Geometry check sheet. Reference: the model listing, model coordinates, mm. Coordinates: 2 decimals unless noted, no trailing zeros. Loops run counter-clockwise (first coordinate to the right, second up) from the corner with the lowest first, then second, coordinate; pieces in that order, holes last. Notation, with made-up numbers: M -21.5,7 L 28.5,7 A9 cw 28.5,24 Z; hole C -4,48.25 d9. An arc over 180 degrees is marked long. Use CSV: the item, a comma, the result in double quotes.
```python
from build123d import *

# Parameters (mm, degrees)
EXTRUDE_1_DEPTH     = 100
SKETCH_2_R          = 1.45
CUT_EXTRUDE_1_DEPTH = 10
SKETCH_3_R          = 1.45
CUT_EXTRUDE_2_DEPTH = 10


with BuildPart() as part:
    # Эскиз1 → Бобышка-Вытянуть1 (new, symmetric)
    with BuildSketch(Plane(origin=(0, 0, 0), x_dir=(0, 0, -1), z_dir=(1, 0, 0))):
        with BuildLine():
            Line((-3.085485457, 17.498657575), (-2.386593122, 13.535042182))
            Line((-2.386593122, 13.535042182), (2.386593122, 13.535042182))
            Line((2.386593122, 13.535042182), (3.085485457, 17.498657575))
            ThreePointArc((3.085485457, 17.498657575), (0, 17.604562424), (-3.085485457, 17.498657575))
        make_face()
    extrude(amount=EXTRUDE_1_DEPTH, both=True)

    # Эскиз2 → Вырез-Вытянуть1 (cut)
    with BuildSketch(Plane(origin=(100, 0, 0), x_dir=(0, 0, -1), z_dir=(1, 0, 0))):
        with Locations((0, 15.604562424)):
            Circle(SKETCH_2_R)
    cut_extrude_1 = extrude(amount=-CUT_EXTRUDE_1_DEPTH, mode=Mode.SUBTRACT)

    # Зеркальное отражение1: Вырез-Вытянуть1 across plane
    add(cut_extrude_1.mirror(Plane(origin=(0, 0, 0), x_dir=(0, 0, 1), z_dir=(1, 0, 0))), mode=Mode.SUBTRACT)

    # Эскиз3 → Вырез-Вытянуть2 (cut)
    with BuildSketch(Plane.XZ.offset(-13.535042182)):
        with Locations(Location((-20, 0, 0), (0, 0, 270))):
            Circle(SKETCH_3_R)
        with Locations(Location((20, 0, 0), (0, 0, 270))):
            Circle(SKETCH_3_R)
    extrude(amount=-CUT_EXTRUDE_2_DEPTH, mode=Mode.SUBTRACT)


solid = part.part
```
1. Section check B-B, the plane x = 35. Record the cut outline in (y, z).
The answers:
outline,"M 13.54,-2.39 L 17.5,-3.09 A45 ccw 17.5,3.09 L 13.54,2.39 Z"
2. Release check for a two-part mould opening along Z. For faces 1 (the flat face through (1.4, 15.54, 2.74)), 2 (the flat face through (1, 13.535, 0)), 3 (the flat face through (1.4, 15.49, -2.73)), 4 (the cylindrical face through (1.4, 17.605, -0.043)) record: +Z half, -Z half, draft (parallel to the pull), parting line (faces both ways), or undercut.
The answers:
face 1,"+Z half"
face 2,"draft"
face 3,"-Z half"
face 4,"parting line"
3. Thickness scan on line 1 (X direction, y = 15.6, z = 0); line 2 (X direction, y = 17.45, z = 1.25); line 3 (Y direction, x = 91, z = 0). Record the ranges inside material, lowest first. Write a range as [from, to].
The answers:
line 1,"[-90, -21.45], [-18.55, 18.55], [21.45, 90]"
line 2,"[-100, -20.73], [-19.27, 19.27], [20.73, 100]"
line 3,"[13.54, 14.15], [17.05, 17.6]"
4. Section check C-C, the plane y = 14.95. Record the cut outline in (x, z), plus the area to 3 significant figures.
The answers:
outline,"M -100,-2.64 L 100,-2.64 L 100,-1.29 L 90,-1.29 L 90,1.29 L 100,1.29 L 100,2.64 L -100,2.64 L -100,1.29 L -90,1.29 L -90,-1.29 L -100,-1.29 Z; hole C -20,0 d2.9; hole C 20,0 d2.9"
area,"989 mm^2"
5. Section check A-A, the plane z = 0. Record the cut outline in (x, y).
The answers:
outline,"M -100,13.54 L -21.45,13.54 L -21.45,17.6 L -100,17.6 L -100,17.05 L -90,17.05 L -90,14.15 L -100,14.15 Z; M -18.55,13.54 L 18.55,13.54 L 18.55,17.6 L -18.55,17.6 Z; M 21.45,13.54 L 100,13.54 L 100,14.15 L 90,14.15 L 90,17.05 L 100,17.05 L 100,17.6 L 21.45,17.6 Z"
